from build123d import *

# Parameters (mm, degrees)
SKETCH_W           = 23.599997
SKETCH_H           = 28.600128
SKETCH_R           = 1.75088
PAD_DEPTH          = 20.5
HOLE_D             = 4.8
HOLE_DEPTH         = 34
HOLE_CBORE_D       = 10
HOLE_CBORE_DEPTH   = 2.02
SKETCH002_W        = 6.496036
SKETCH002_H        = 19.001464
POCKET_DEPTH       = 19
POCKET001_DEPTH    = 19
POCKET001_FACE20_W = 6.501685
POCKET001_FACE20_H = 19
POCKET002_DEPTH    = 40
POCKET003_DEPTH    = 3.3
POCKET004_DEPTH    = 5
POCKET004_FACE5_W  = 20.5
POCKET004_FACE5_H  = 28.600128
POCKET005_DEPTH    = 2
POCKET006_DEPTH    = 20


with BuildPart() as part:
    # Sketch → Pad (new body)
    with BuildSketch(Plane.XZ):
        with Locations((0.4742105, 393.081741)):
            Rectangle(SKETCH_W, SKETCH_H)
        with Locations((2.474405, 393.078932)):
            Circle(SKETCH_R, mode=Mode.SUBTRACT)
    extrude(amount=-PAD_DEPTH)

    # Hole
    with Locations(Plane.XY.offset(407.4)):
        with Locations((0.346603, 14.950747)):
            CounterBoreHole(HOLE_D / 2, HOLE_CBORE_D / 2, HOLE_CBORE_DEPTH, depth=HOLE_DEPTH)

    # Sketch002 → Pocket (cut)
    with BuildSketch(Plane.YZ.offset(-3.5)):
        with Locations((7.252294, 393.082428)):
            Rectangle(SKETCH002_W, SKETCH002_H)
    extrude(amount=POCKET_DEPTH, mode=Mode.SUBTRACT)

    # Sketch003 → Pocket001 (cut)
    with BuildSketch(Plane.XY.offset(383.58)):
        with BuildLine():
            ThreePointArc((-8.5264420268, 9.000709), (-7.0612425813, 5.4638025679), (-3.5244, 3.998449))
            Line((-3.5244, 3.998449), (-3.5244, 10.500134))
            Line((-3.5244, 10.500134), (4.225286, 10.500134))
            Line((4.225286, 10.500134), (4.225286, 24.874678))
            Line((4.225286, 24.874678), (-8.5264420268, 21.309877))
            Line((-8.5264420268, 9.000709), (-8.5264420268, 21.309877))
        make_face()
    extrude(amount=POCKET001_DEPTH, mode=Mode.SUBTRACT)

    # Pocket001 Face20 → Pocket002 (cut)
    with BuildSketch(Plane(origin=(-3.5244, 7.2492915, 393.08), x_dir=(0, 1, 0), z_dir=(-1, 0, 0))):
        Rectangle(POCKET001_FACE20_W, POCKET001_FACE20_H)
    extrude(amount=-POCKET002_DEPTH, mode=Mode.SUBTRACT)

    # Sketch004 → Pocket003 (cut)
    with BuildSketch(Plane.XZ.offset(-4)):
        Polygon((0.857594, 395.881653), (-0.7589761165, 393.0817985758), (0.8574838835, 390.2818805758), (4.090514, 390.281817), (5.7070841165, 393.0816714242), (4.0906241165, 395.8815894242), align=None)
    extrude(amount=POCKET003_DEPTH, mode=Mode.SUBTRACT)

    # Pocket003 Face12 → Pocket004 (cut)
    with BuildSketch(Plane(origin=(4.225286, 15.5001559921, 393.0799999849), x_dir=(0, 1, 0), z_dir=(-1, 0, 0))):
        Polygon((4.9998440079, 9.4999999849), (-5.0000219921, 9.4999999849), (-5.0000219921, 9.4983039849), (-4.9998439921, 9.4983039849), (-4.9998439921, -9.5000000151), (4.9998440079, -9.5000000151), align=None)
    extrude(amount=-POCKET004_DEPTH, mode=Mode.SUBTRACT)

    # Pocket004 Face5 → Pocket005 (cut)
    with BuildSketch(Plane(origin=(12.274209, 11.051181849, 393.0817843597), x_dir=(0, -1, 0), z_dir=(1, 0, 0))):
        with Locations((0.801181849, 4.33597e-05)):
            Rectangle(POCKET004_FACE5_W, POCKET004_FACE5_H)
        Polygon((7.046905849, -9.5013756403), (0.550869849, -9.5013756403), (0.550869849, 9.5000883597), (0.551047849, 9.5000883597), (0.551047849, 9.5017843597), (7.052732849, 9.5017843597), (7.052732849, -9.4982156403), (7.046905849, -9.4982156403), align=None, mode=Mode.SUBTRACT)
    extrude(amount=-POCKET005_DEPTH, mode=Mode.SUBTRACT)

    # Pocket005 Face10 → Pocket006 (cut)
    with BuildSketch(Plane(origin=(9.7358804108, 10.500312, 393.1015544105), x_dir=(-1, 0, 0), z_dir=(0, -1, 0))):
        Polygon((13.2358804108, -9.4816055895), (13.2358804108, -9.4784455895), (0.5105944108, -9.4784455895), (0.5105944108, 9.5198584105), (-0.5383285892, 9.5198584105), (-0.5383285892, -9.4816055895), align=None)
    extrude(amount=-POCKET006_DEPTH, mode=Mode.SUBTRACT)


solid = part.part
The model under review builds one solid part; all positions refer to its coordinate system, in mm. A direction names the side the tool comes from. Give positions to 0.01 mm unless a question says otherwise; leave off trailing zeros. Loops run counter-clockwise (first coordinate to the right, second up) from the corner with the lowest first, then second, coordinate; pieces in that order, holes last. Notation, with made-up numbers: (80.25, 43) -> (130.25, 43) arc R14 cw to (130.25, 56) -> close; hole circle Ø2 at (56, 81.25). An arc over 180 degrees is marked (long way). Put each result on its own line as item: value. Start each with the question number.
1. Wall thickness on probe 1 along Z at (x, y) = (-7.5, 18); probe 2 along Z at (x, y) = (2.5, 1); probe 3 along Y at (x, z) = (-3.25, 388.5): over which ranges is each line inside the solid? List them lowest first.
2. We need section C-C on z = 394. State the section outline as (x, y) points.
3. We need section D-D on z = 388. State the section outline as (x, y) points, then the cut area to 3 significant figures.
4. For faces 1 (the face through (-0.74, 10.07, 406.39)), 2 (the face through (10.274, 3.6, 389.7)), 3 (the face through (0.04, 2.37, 391.7)), 4 (the face through (10, 15, 383.582)), list the 3-axis set-ups (+Z, -Z, +X, -X, +Y, -Y) from which the entire face can be reached by the end or side of a thin tool; tool diameter is ignored.
5. Mouldability with a two-part tool opening along Z and no side actions: class faces 5 (the face through (-2, 16, 405.38)), 6 (the face through (4.91, 2.37, 394.46)), 7 (the face through (-3, 20.5, 403)) as released by +Z, released by -Z, zero draft, split by the parting line, or undercut.
6. We need section A-A on y = 15.75. State how many separate pieces and enclosed holes the cut face has, then the cut area to 3 significant figures.
7. Clearance check with flat-ended pins moving along their axes: P1, Ø1.7, axis at x = 1, z = 394.5, coming from the +Y side; P2, Ø10, axis at x = -2, z = 391.5, coming from the +Y side; P3, Ø9, axis at y = 13, z = 392, coming from the +X side. State where each tip first meets the part, or that it passes through.
Determined:
1. probe 1: 378.78 to 383.58, 402.58 to 407.38
1. probe 2: 378.78 to 390.28, 395.88 to 407.38
1. probe 3: 0 to 4
2. outline: (-11.33, 0) -> (0.99, 0) -> (0.99, 0.7) -> (-0.23, 0.7) -> (-0.23, 4) -> (-3.52, 4) arc R5 cw to (-8.53, 9) -> (-8.53, 20.5) -> (-11.33, 20.5) -> close; (3.96, 0) -> (10.27, 0) -> (10.27, 4) -> (5.18, 4) -> (5.18, 0.7) -> (3.96, 0.7) -> close
3. outline: (-11.33, 0) -> (10.27, 0) -> (10.27, 4) -> (-3.52, 4) arc R5 cw to (-8.53, 9) -> (-8.53, 20.5) -> (-11.33, 20.5) -> close
3. area: 138 mm^2
4. face 1: +Z
4. face 2: +Z, -Z, +X, +Y, -Y
4. face 3: +Y
4. face 4: +X, +Y
5. face 5: released by +Z
5. face 6: undercut
5. face 7: zero draft
6. separate pieces: 3
6. enclosed holes: 0
6. area: 206 mm^2
7. P1: y = 4
7. P2: y = 5.4
7. P3: x = -8.5
